For this review, use the dimensioned drawing (mm, ordinates from the lowest corner) and the shaded views. A direction names the side the tool comes from. Coordinates: 2 decimals unless noted, no trailing zeros. Loops run counter-clockwise (first coordinate to the right, second up) from the corner with the lowest first, then second, coordinate; pieces in that order, holes last. Notation, with made-up numbers: M 25,76.5 L 45,76.5 A27 ccw 45,95.5 Z; hole C 4,55.25 d3. An arc over 180 degrees is marked long. Write item = value, one per line. Start each with the question number.
Q1. We need section A-A on x = 6. Give the boundary of the cut face in (y, z).
Q2. Mouldability with a two-part tool opening along X and no side actions: class the marked faces 1, 2 and 3 as released by +X, released by -X, zero draft, split by the parting line, or undercut.
Q3. We need section D-D on y = 9.25. Give the boundary of the cut face in (x, z).
Q4. We need section B-B on y = 5. Give the boundary of the cut face in (x, z).
Q5. For the marked faces 4, 5 and 6, list the 3-axis set-ups (+Z, -Z, +X, -X, +Y, -Y) from which the entire face can be reached by the end or side of a thin tool; tool diameter is ignored.
Q6. Clearance check with flat-ended pins moving along their axes: pin 1 Ø8 at (y, z) = (3.5, 18.5) entering from +X; pin 2 Ø5 at (x, z) = (17.5, 18.5) entering from +Y; pin 3 Ø5 at (y, z) = (13.5, 15) entering from +X; pin 4 Ø4 at (x, y) = (27.64, 16.64) entering from +Z. State where each tip first meets the part, or that it passes through.
Q7. We need section C-C on z = 9.75. Give the boundary of the cut face in (x, y) (1 decimal), and give its area (3 significant figures).
Q8. Wall thickness on probe 1 along Y at (x, z) = (6, 13.25); probe 2 along Z at (x, y) = (29, 15.5); probe 3 along Y at (x, z) = (10, 18.5): over which ranges is each line inside the solid? List them lowest first.
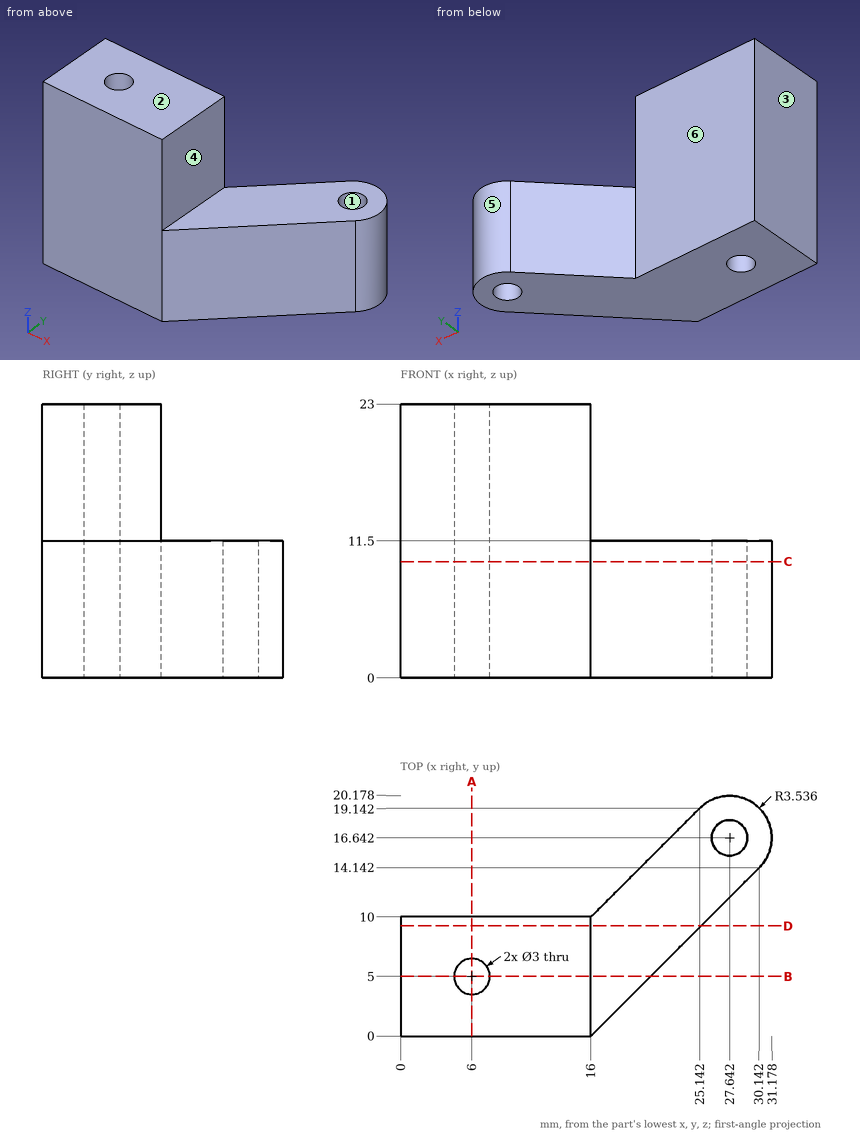
Returned:
q1.outline = M 0,0 L 3.5,0 L 3.5,23 L 0,23 Z; M 6.5,0 L 10,0 L 10,23 L 6.5,23 Z
q2.face_1 = undercut
q2.face_2 = zero draft
q2.face_3 = released by -X
q3.outline = M 0,0 L 25.25,0 L 25.25,11.5 L 16,11.5 L 16,23 L 0,23 Z
q4.outline = M 0,0 L 4.5,0 L 4.5,23 L 0,23 Z; M 7.5,0 L 21,0 L 21,11.5 L 16,11.5 L 16,23 L 7.5,23 Z
q5.face_4 = +Z, +X, +Y, -Y
q5.face_5 = +Z, -Z
q5.face_6 = +Z, -Z, -X, +Y
q6.pin_1 = 16
q6.pin_2 = 10
q6.pin_3 = through
q6.pin_4 = 11.5
q7.outline = M 0,0 L 16,0 L 30.1,14.1 A3.5 ccw 25.1,19.1 L 16,10 L 0,10 Z; hole C 6,5 d3; hole C 27.6,16.6 d3
q7.area = 282 mm^2
q8.probe_1 = 0 to 3.5, 6.5 to 10
q8.probe_2 = 0 to 11.5
q8.probe_3 = 0 to 10
